Check sheet for the drawn part. Datum: minimum x, y, z corner. Units: mm. Round coordinates to 2 decimals unless told otherwise and drop trailing zeros. Order: outer loops, then holes, each group sorted by start corner. A loop starts at its lowest first (then second) coordinate and runs counter-clockwise, first axis right, second up.
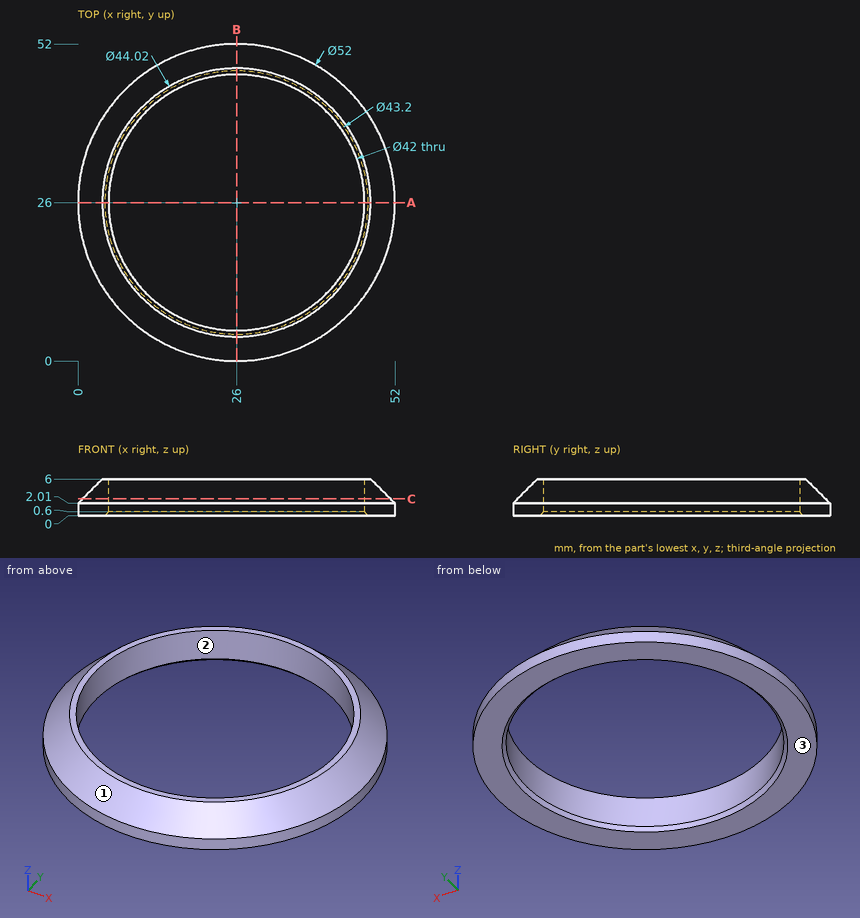
1) Sectioned sample at A-A on y = 26. Record the cut outline in (x, z), and give its area (3 significant figures).
2) Draft check along X on the marked faces 1, 2 and 3. Enter one of: pulls with the +X half, pulls with the -X half, needs draft (parallel to the pull), parting line crosses it, or undercut.
3) Sectioned sample at C-C on z = 2.75. Record the cut outline in (x, y).
4) Gauge pin test, flat ends, axial feed: pin 1 (1 mm diameter, centred on y = 5.5, z = 3.5, fed in from +X); pin 2 (2 mm diameter, centred on y = 43.5, z = 5, fed in from -X); pin 3 (1.5 mm diameter, centred on y = 19.5, z = 3.5, fed in from +X). Record the tip position at first contact, or that the pin passes through.
5) Scan lines: line 1 (Y direction, x = 39, z = 4.05); line 2 (Z direction, x = 45, y = 40); line 3 (X direction, y = 37, z = 2.2). Record each from-to range of solid material in increasing order.
Values found:
1. outline: (0, 0) - (4.4, 0) - (5, 0.6) - (5, 6) - (3.99, 6) - (0, 2.01) - close; (47, 0.6) - (47.6, 0) - (52, 0) - (52, 2.01) - (48.01, 6) - (47, 6) - close
1. area: 43.7 mm2
2. face 1: parting line crosses it
2. face 2: undercut
2. face 3: needs draft
3. outline: circle Ø50.52 at (26, 26); hole circle Ø42 at (26, 26)
4. pin 1: stops at x = 40.58
4. pin 2: stops at x = 9.23
4. pin 3: stops at x = 50.43
5. line 1: y = 5.87 to 9.51, 42.49 to 46.13
5. line 2: z = 0 to 4.41
5. line 3: x = 2.65 to 8.11, 43.89 to 49.35
